Part print with two shaded views. Sizes in mm from the minimum x, y, z corner. A direction names the side the tool comes from. Coordinates: 2 decimals unless noted, no trailing zeros.
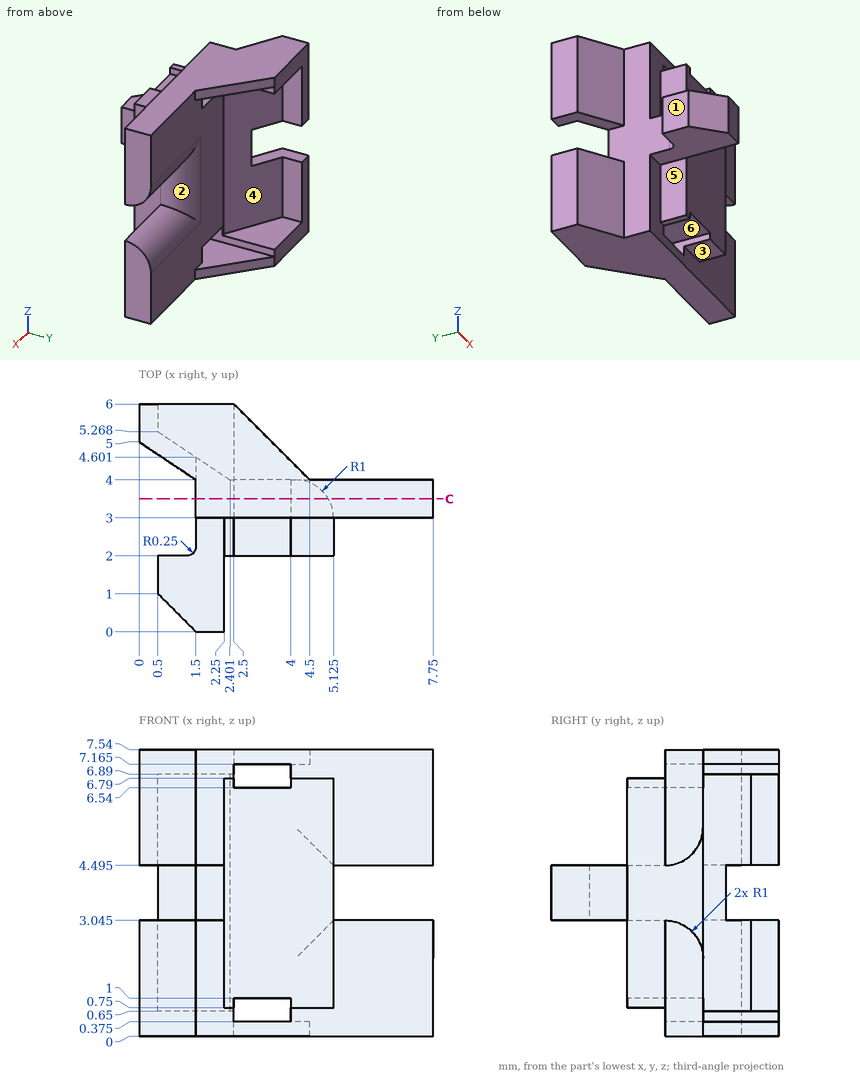
Q1. Cut at C-C on y = 3.5. Count the separate pieces of the cut face and the enclosed holes in it, and give its area (3 significant figures).
Results list:
separate pieces: 1
enclosed holes: 2
area: 40.5 mm2
Q2. Pin check, flat tips, straight feed: pin 1 Ø2 at (y, z) = (5, 5.5) entering from -X; pin 2 Ø1.5 at (x, z) = (3.5, 2) entering from -Y; pin 3 Ø1.2 at (y, z) = (4, 3.5) entering from -X (1 decimal); pin 4 Ø0.8 at (y, z) = (2.5, 5.5) entering from -X. Stop position of each tip, or through.
Results list:
pin 1: stops at x = 0
pin 2: stops at y = 2
pin 3: stops at x = 0.9
pin 4: stops at x = 2.25
Q3. Wall check: line 1 along X through (y, z) = (3.25, 0.75); line 2 along Z through (x, y) = (1.5, 5.6); line 3 along X through (y, z) = (5.75, 6.25). Give the ranges that are in metal, low to high.
Results list:
line 1: x = 1.5 to 2.5, 4 to 7.75
line 2: z = 0 to 0.65, 6.89 to 7.54
line 3: x = 0 to 0.5
Q4. Mould opens along Z. For the marked faces 1, 2 and 3 say: pulls with the +Z half, pulls with the -Z half, needs draft (parallel to the pull), parting line crosses it, or undercut.
Results list:
face 1: needs draft
face 2: undercut
face 3: pulls with the -Z half
Q5. Which spindle directions (+Z, -Z, +X, -X, +Y, -Y) get a long thin tool onto all of the face, cutting with end or side? Do the marked faces 4, 5 and 6. Say none if no direction does.
Results list:
face 4: +X, +Y
face 5: -Z, -X, -Y
face 6: +Y, -Y
